Work out the finished part from the listing and answer in its coordinate system (mm). Round coordinates to 2 decimals unless told otherwise and drop trailing zeros. Order: outer loops, then holes, each group sorted by start corner. A loop starts at its lowest first (then second) coordinate and runs counter-clockwise, first axis right, second up. Notation, with made-up numbers: (-39.5, 48.25) - (3.5, 48.25) arc R21 ccw to (3.5, 62.25) - close; hole circle Ø6 at (75, 80). An arc over 180 degrees is marked (long way). One line per question, with ' | ' between items. Start each with the question number.
from build123d import *

# Parameters (mm, degrees)
PAD005_DEPTH    = 2.5
CHAMFER003_SIZE = 1


with BuildPart() as obj1:
    # Sketch → Pad005 (new body, symmetric)
    with BuildSketch(Plane.XY):
        Polygon((37.36659, 29.932996), (43.095788, 29.268148), (41.474087, 23.988274), (37.214632, 24.991065), align=None)
    extrude(amount=PAD005_DEPTH, both=True)

    # Chamfer003
    chamfer003_edges = [obj1.edges().sort_by_distance(p)[0] for p in [
        (42.284938, 26.628211, 2.5),
        (37.290611, 27.46203, 2.5),
        (42.284938, 26.628211, -2.5),
        (37.290611, 27.46203, -2.5),
    ]]
    chamfer(chamfer003_edges, length=CHAMFER003_SIZE)


with BuildPart() as part_mirroring001:
    # Part__Mirroring001: instance of obj1
    add(obj1.part.mirror(Plane(origin=(0, 0, 0), x_dir=(0, -1, 0), z_dir=(1, 0, 0))))


solid = part_mirroring001.part
1) Section B-B on z = -0.6 is taken. Give the vertices of the cut face in (x, y), and give its area (3 significant figures).
2) Section A-A on y = 26.3 is taken. Give the vertices of the cut face in (x, z).
3) Flat-ended cylindrical pins translate along their axes: pin 1 (3 mm diameter, centred on x = -42.5, y = 27.5, fed in from -Z); pin 2 (2 mm diameter, centred on x = -40, z = 1.5, fed in from -Y); pin 3 (1 mm diameter, centred on y = 27.5, z = 1.5, fed in from -X). Find the tip coordinate at first contact, or state that the pin passes through.
4) Section D-D on y = 29.1 is taken. Give the vertices of the cut face in (x, z), and give its area (3 significant figures).
5) Section C-C on x = -38.8 is taken. Give the vertices of the cut face in (y, z).
6) Straight lines are drawn through the part: line 1 (X direction, y = 27, z = 1.8); line 2 (X direction, y = 25.75, z = -0.5); line 3 (Y direction, x = -37.85, z = -1.3). For each, find the intervals that lie inside material, in ascending order.
7) Determine the mould class of faces 1 (the flat face through (-40, 27, 2.5)), 2 (the flat face through (-41.8, 26.78, -2.01)), 3 (the flat face through (-40.191, 29.605, 0.035)) for opening direction Z: released by +Z, released by -Z, zero draft, split by the parting line, or undercut.
Recorded:
1) outline: (-43.1, 29.27) - (-41.47, 23.99) - (-37.21, 24.99) - (-37.37, 29.93) - close | area: 26.3 mm²
2) outline: (-42.18, -1.5) - (-41.14, -2.5) - (-38.26, -2.5) - (-37.25, -1.5) - (-37.25, 1.5) - (-38.26, 2.5) - (-41.14, 2.5) - (-42.18, 1.5) - close
3) pin 1: stops at z = -2.5 | pin 2: stops at y = 24.1 | pin 3: stops at x = -42.71
4) outline: (-43.04, -1.5) - (-42, -2.5) - (-38.34, -2.5) - (-37.34, -1.5) - (-37.34, 1.5) - (-38.34, 2.5) - (-42, 2.5) - (-43.04, 1.5) - close | area: 26.5 mm²
5) outline: (24.62, -2.5) - (29.77, -2.5) - (29.77, 2.5) - (24.62, 2.5) - close
6) line 1: x = -42.09 to -37.58 | line 2: x = -42.02 to -37.24 | line 3: y = 24.84 to 29.88
7) face 1: released by +Z | face 2: released by -Z | face 3: zero draft
